```python
from build123d import *

# Parameters (mm, degrees)
SKETCH_1_R          = 20
EXTRUDE_1_DEPTH     = 2.2
SKETCH_2_R          = 18.5
EXTRUDE_2_DEPTH     = 6.8
SKETCH_3_R          = 10
CUT_EXTRUDE_1_DEPTH = 9
SKETCH_4_R          = 17
SKETCH_4_R_2        = 12
CUT_EXTRUDE_2_DEPTH = 0.5
CUT_EXTRUDE_START   = -0.5
SKETCH_5_R          = 17
SKETCH_5_R_2        = 12
CUT_EXTRUDE_3_DEPTH = 0.5


with BuildPart() as part:
    # 草图1 → 凸台-拉伸1 (new body)
    with BuildSketch(Plane(origin=(0, 0, 0), x_dir=(1, 0, 0), z_dir=(0, 1, 0))):
        with Locations(Location((0, 0, 0), (0, 0, 270))):
            Circle(SKETCH_1_R)
    extrude(amount=EXTRUDE_1_DEPTH)

    # 草图2 → 凸台-拉伸2 (add)
    with BuildSketch(Plane(origin=(0, 2.2, 0), x_dir=(1, 0, 0), z_dir=(0, 1, 0))):
        with Locations(Location((0, 0, 0), (0, 0, 270))):
            Circle(SKETCH_2_R)
    extrude(amount=EXTRUDE_2_DEPTH)

    # 草图3 → 切除-拉伸1 (cut)
    with BuildSketch(Plane(origin=(0, 9, 0), x_dir=(1, 0, 0), z_dir=(0, 1, 0))):
        with Locations(Location((0, 0, 0), (0, 0, 270))):
            Circle(SKETCH_3_R)
    extrude(amount=-CUT_EXTRUDE_1_DEPTH, mode=Mode.SUBTRACT)

    # 草图4 → 切除-拉伸2 (cut)
    with BuildSketch(Plane.XZ):
        with Locations(Location((0, 0, 0), (0, 0, 270))):
            Circle(SKETCH_4_R)
        with Locations(Location((0, 0, 0), (0, 0, 270))):
            Circle(SKETCH_4_R_2, mode=Mode.SUBTRACT)
    extrude(amount=-CUT_EXTRUDE_2_DEPTH, mode=Mode.SUBTRACT)

    # 草图5 → 切除-拉伸3 (cut)
    with BuildSketch(Plane(origin=(0, 9, 0), x_dir=(1, 0, 0), z_dir=(0, 1, 0)).offset(CUT_EXTRUDE_START)):
        with Locations(Location((0, 0, 0), (0, 0, 90))):
            Circle(SKETCH_5_R)
        with Locations(Location((0, 0, 0), (0, 0, 90))):
            Circle(SKETCH_5_R_2, mode=Mode.SUBTRACT)
    extrude(amount=CUT_EXTRUDE_3_DEPTH, mode=Mode.SUBTRACT)


solid = part.part
```
CAD build for the part. Positions are in the model's coordinates, mm. A direction names the side the tool comes from. Round coordinates to 2 decimals unless told otherwise and drop trailing zeros. Order: outer loops, then holes, each group sorted by start corner. A loop starts at its lowest first (then second) coordinate and runs counter-clockwise, first axis right, second up.
Item 1: Probe line 1 along X through (y, z) = (8.9, 0); line 2 along X through (y, z) = (0.2, 0); line 3 along X through (y, z) = (2.5, 0). List the from-to ranges inside material, lowest first.
Item 2: Saw through at B-B on z = 0. Write the cut outline in (x, y).
Item 3: Saw through at C-C on y = 3. Write the cut outline in (x, z), then the cut area to 3 significant figures.
Item 4: Tool access for faces 1 (the face through (4, 8.5, 12)), 2 (the face through (9, 9, -5)), 3 (the face through (-4, 0.5, 12)): list every direction of +Z, -Z, +X, -X, +Y, -Y with a clear straight run to the whole face (end or side of a thin tool).
Item 5: Mould opens along X. For faces 4 (the face through (-18, 2.2, 6)), 5 (the face through (-7.086, 5.552, 17.089)), 6 (the face through (16.855, 0.246, 2.213)) say: pulls with the +X half, pulls with the -X half, needs draft (parallel to the pull), parting line crosses it, or undercut.
Item 6: Pin check, flat tips, straight feed: pin 1 (4 mm diameter, centred on x = -4.5, y = 2.5, fed in from -Z); pin 2 (2 mm diameter, centred on x = -13, y = 2.5, fed in from -Z). Stop position of each tip, or through.
Item 7: Saw through at A-A on x = 0. Write the cut outline in (y, z).
Item 8: Saw through at D-D on x = -15. Write the cut outline in (y, z), then the cut area to 3 significant figures.
Reported:
1. line 1: x = -18.5 to -17, -12 to -10, 10 to 12, 17 to 18.5
1. line 2: x = -20 to -17, -12 to -10, 10 to 12, 17 to 20
1. line 3: x = -18.5 to -10, 10 to 18.5
2. outline: (-20, 0) - (-17, 0) - (-17, 0.5) - (-12, 0.5) - (-12, 0) - (-10, 0) - (-10, 9) - (-12, 9) - (-12, 8.5) - (-17, 8.5) - (-17, 9) - (-18.5, 9) - (-18.5, 2.2) - (-20, 2.2) - close; (10, 0) - (12, 0) - (12, 0.5) - (17, 0.5) - (17, 0) - (20, 0) - (20, 2.2) - (18.5, 2.2) - (18.5, 9) - (17, 9) - (17, 8.5) - (12, 8.5) - (12, 9) - (10, 9) - close
3. outline: circle Ø37 at (0, 0); hole circle Ø20 at (0, 0)
3. area: 761 mm2
4. face 1: +Y
4. face 2: +Z, -Z, +X, -X, +Y
4. face 3: -Y
5. face 4: needs draft
5. face 5: parting line crosses it
5. face 6: undercut
6. pin 1: stops at z = -19.84
6. pin 2: stops at z = -15.97
7. outline: (0, -20) - (2.2, -20) - (2.2, -18.5) - (9, -18.5) - (9, -17) - (8.5, -17) - (8.5, -12) - (9, -12) - (9, -10) - (0, -10) - (0, -12) - (0.5, -12) - (0.5, -17) - (0, -17) - close; (0, 10) - (9, 10) - (9, 12) - (8.5, 12) - (8.5, 17) - (9, 17) - (9, 18.5) - (2.2, 18.5) - (2.2, 20) - (0, 20) - (0, 17) - (0.5, 17) - (0.5, 12) - (0, 12) - close
8. outline: (0, -13.23) - (2.2, -13.23) - (2.2, -10.83) - (9, -10.83) - (9, -8) - (8.5, -8) - (8.5, 8) - (9, 8) - (9, 10.83) - (2.2, 10.83) - (2.2, 13.23) - (0, 13.23) - (0, 8) - (0.5, 8) - (0.5, -8) - (0, -8) - close
8. area: 189 mm2
